from build123d import *

# Parameters (mm, degrees)
BOSS_EXTRUDE1_DEPTH        = 3.556
BOSS_EXTRUDE1_DEPTH_BACK   = 3.556
F_3_4_0_4_DIAMETER_HOLE1_D = 10.16


with BuildPart() as part:
    # Sketch1 → Boss-Extrude1 (new, two sides: drawn at the far end of the back side and taken through both)
    with BuildSketch(Plane.XY.offset(-BOSS_EXTRUDE1_DEPTH_BACK)):
        with BuildLine():
            Line((46.336307345, 120.396), (46.336307345, 15.24))
            Line((46.336307345, 15.24), (-55.263692655, 15.24))
            Line((-55.263692655, 15.24), (-165.807846327, 125.784153673))
            ThreePointArc((-165.807846327, 125.784153673), (-176.584153673, 125.784153673), (-176.584153673, 115.007846327))
            Line((-176.584153673, 115.007846327), (-61.576307345, 0))
            Line((-61.576307345, 0), (61.576307345, 0))
            Line((61.576307345, 0), (61.576307345, 120.396))
            ThreePointArc((61.576307345, 120.396), (53.956307345, 128.016), (46.336307345, 120.396))
        make_face()
    extrude(amount=BOSS_EXTRUDE1_DEPTH + BOSS_EXTRUDE1_DEPTH_BACK)

    # 3/4 (0.4) Diameter Hole1 (through all)
    with Locations(Plane.XY.offset(3.556)):
        with Locations((-171.196, 120.396), (53.956307345, 120.396)):
            Hole(F_3_4_0_4_DIAMETER_HOLE1_D / 2)


solid = part.part
Check sheet for the modelled part. Datum: model origin and axes. Units: mm. A direction names the side the tool comes from. Round coordinates to 2 decimals unless told otherwise and drop trailing zeros. Write each loop counter-clockwise with the first axis right and the second up, starting at its lowest first coordinate (ties: lowest second). Pieces come first, ordered by that corner, then holes. Notation, with made-up numbers: (-3, -18.75) - (36, -18.75) arc R36 ccw to (36, 20.25) - close; hole circle Ø11 at (46, 46). An arc over 180 degrees is marked (long way). Return JSON: item names as keys, results as strings.
Q1. Access from +Z, -Z, +X, -X, +Y, -Y to the whole of each face (thin tool, end or side, straight path). Record for faces 1 (the cylindrical face through (55.058, 115.437, -0.05)), 2 (the flat face through (-109.762, 69.738, -0.05)).
Returned:
{"face 1": "+Z, -Z", "face 2": "+Z, -Z, +Y"}
Q2. Draft check along X on faces 3 (the flat face through (-119.885, 58.309, -0.05)), 4 (the flat face through (-1, 0, 0)), 5 (the cylindrical face through (-176.464, 125.901, -0.05)). Enter one of: released by +X, released by -X, zero draft, split by the parting line, or undercut.
Returned:
{"face 3": "released by -X", "face 4": "zero draft", "face 5": "undercut"}
Q3. Cross-section at A-A (z = -0.75). Record the boundary of the cut face in (x, y), then the cut area to 3 significant figures.
Returned:
{"outline": "(-176.58, 115.01) - (-61.58, 0) - (61.58, 0) - (61.58, 120.4) arc R7.62 ccw to (46.34, 120.4) - (46.34, 15.24) - (-55.26, 15.24) - (-165.81, 125.78) arc R7.62 ccw to start; hole circle Ø10.16 at (-171.2, 120.4); hole circle Ø10.16 at (53.96, 120.4)", "area": "5,880 mm²"}
Q4. Scan lines: L1, parallel to Y at x = 20.5, z = -1.5; L2, parallel to X at y = 58, z = 0.75; L3, parallel to X at y = 87, z = 2. Record each from-to range of solid material in increasing order. Write a range as from..to.
Returned:
{"L1": "y = 0..15.24", "L2": "x = -119.58..-98.02, 46.34..61.58", "L3": "x = -148.58..-127.02, 46.34..61.58"}
Q5. Depth check by flat-ended pin: P1, Ø1, axis at x = -76, z = -1, coming from the +Y side; P2, Ø4, axis at y = 14, z = 2, coming from the -X side. Enter the tip coordinate at first touch or a pass-through.
Returned:
{"P1": "stops at y = 36.48", "P2": "stops at x = -77.58"}
Q6. Cross-section at D-D (x = -139). Record the boundary of the cut face in (y, z), then the cut area to 3 significant figures.
Returned:
{"outline": "(77.42, -3.56) - (98.98, -3.56) - (98.98, 3.56) - (77.42, 3.56) - close", "area": "153 mm²"}
Q7. Cross-section at B-B (y = 30). Record the boundary of the cut face in (x, z).
Returned:
{"outline": "(-91.58, -3.56) - (-70.02, -3.56) - (-70.02, 3.56) - (-91.58, 3.56) - close; (46.34, -3.56) - (61.58, -3.56) - (61.58, 3.56) - (46.34, 3.56) - close"}
Q8. Cross-section at C-C (x = -6.5). Record the boundary of the cut face in (y, z), then the cut area to 3 significant figures.
Returned:
{"outline": "(0, -3.56) - (15.24, -3.56) - (15.24, 3.56) - (0, 3.56) - close", "area": "108 mm²"}
